Could you check a few things on this model? Use its own coordinates, in mm. A direction names the side the tool comes from. Round coordinates to 2 decimals unless told otherwise and drop trailing zeros. Loops run counter-clockwise (first coordinate to the right, second up) from the corner with the lowest first, then second, coordinate; pieces in that order, holes last. Notation, with made-up numbers: (14, 8.25) - (35, 8.25) arc R13 ccw to (35, 23.25) - close; hole circle Ø1 at (9, -32.5). An arc over 180 degrees is marked (long way). Use one line per item in the form item = value.
```python
from build123d import *

# Parameters (mm, degrees)
SKETCH1_W                    = 300
SKETCH1_H                    = 220
BOSS_EXTRUDE1_DEPTH          = 5
SKETCH2_R                    = 12.5
CUT_EXTRUDE1_DEPTH           = 1
F_6_0_6_DIAMETER_HOLE1_D     = 6
F_6_0_6_DIAMETER_HOLE1_DEPTH = 10
F_6_0_6_DIAMETER_HOLE1_TIP   = 1.802581857


with BuildPart() as part:
    # Sketch1 → Boss-Extrude1 (new body)
    with BuildSketch(Plane(origin=(0, 0, 0), x_dir=(1, 0, 0), z_dir=(0, 1, 0))):
        Rectangle(SKETCH1_W, SKETCH1_H)
    extrude(amount=BOSS_EXTRUDE1_DEPTH)

    # Sketch2 → Cut-Extrude1 (cut)
    with BuildSketch(Plane.XZ):
        with Locations(Location((-55, 0, 0), (0, 0, 270))):
            Circle(SKETCH2_R)
    extrude(amount=-CUT_EXTRUDE1_DEPTH, mode=Mode.SUBTRACT)

    # Ø6.0 (6) Diameter Hole1
    with Locations(Plane(origin=(0, 0, 0), x_dir=(-1, 0, 0), z_dir=(0, -1, 0))):
        with Locations((137.5, -97.5), (137.5, 97.5), (-137.5, 97.5), (-137.5, -97.5)):
            Hole(F_6_0_6_DIAMETER_HOLE1_D / 2, depth=F_6_0_6_DIAMETER_HOLE1_DEPTH)
            with Locations((0, 0, -(F_6_0_6_DIAMETER_HOLE1_DEPTH + F_6_0_6_DIAMETER_HOLE1_TIP / 2))):  # 118° drill point
                Cone(0, F_6_0_6_DIAMETER_HOLE1_D / 2, F_6_0_6_DIAMETER_HOLE1_TIP, mode=Mode.SUBTRACT)


solid = part.part
```
1. If we section it at A-A, the plane z = -97.5: Write out the boundary of the cut face in (x, y).
Solution:
outline = (-150, 0) - (-140.5, 0) - (-140.5, 5) - (-150, 5) - close; (-134.5, 0) - (134.5, 0) - (134.5, 5) - (-134.5, 5) - close; (140.5, 0) - (150, 0) - (150, 5) - (140.5, 5) - close
2. If we section it at B-B, the plane x = -137.5: Write out the boundary of the cut face in (y, z).
Solution:
outline = (0, -110) - (5, -110) - (5, -100.5) - (0, -100.5) - close; (0, -94.5) - (5, -94.5) - (5, 94.5) - (0, 94.5) - close; (0, 100.5) - (5, 100.5) - (5, 110) - (0, 110) - close
3. If we section it at C-C, the plane z = 0: Write out the boundary of the cut face in (x, y), plus the area to 4 significant figures.
Solution:
outline = (-150, 0) - (-67.5, 0) - (-67.5, 1) - (-42.5, 1) - (-42.5, 0) - (150, 0) - (150, 5) - (-150, 5) - close
area = 1,475 mm^2
4. We'd pull the mould along X, two halves only. Please class faces 3 (the face through (-42.606, 0.493, 1.627)), 4 (the face through (-136.116, 2.535, -94.838)), 5 (the face through (-2, 0, -2)): +X half, -X half, draft (parallel to the pull), parting line (faces both ways), or undercut.
Solution:
face_3 = undercut
face_4 = undercut
face_5 = draft
5. Please list where these lines run through material, in increasing order: line 1 along Z through (x, y) = (-137.5, 2.85); line 2 along X through (y, z) = (2.1, -97.5); line 3 along X through (y, z) = (0.3, -96).
Solution:
line_1 = -110 to -100.5, -94.5 to 94.5, 100.5 to 110
line_2 = -150 to -140.5, -134.5 to 134.5, 140.5 to 150
line_3 = -150 to -140.1, -134.9 to 134.9, 140.1 to 150
6. For P1, Ø7.5, axis at x = -53, z = 2, coming from the -Y side, with a flat end and sliding along its axis, tell me the tip position at first contact or that it passes through.
Solution:
P1 = 1
7. On a 3-axis mill with a long thin cutter (end or side, diameter ignored), from which of +Z, -Z, +X, -X, +Y, -Y can I reach the whole of each face in a straight line? I mean faces 1 (the face through (-55, 1, 0)), 2 (the face through (-136.116, 2.535, 100.162)). Say none if no direction works.
Solution:
face_1 = -Y
face_2 = +Y, -Y
